The listing builds one solid part. Answer for the finished solid, in the listing's coordinates (mm). A direction names the side the tool comes from. Coordinates: 2 decimals unless noted, no trailing zeros. Order: outer loops, then holes, each group sorted by start corner. A loop starts at its lowest first (then second) coordinate and runs counter-clockwise, first axis right, second up. Notation, with made-up numbers: (54, 45) -> (59, 45) arc R35 ccw to (59, 79) -> close; hole circle Ø1 at (35, 3). An arc over 180 degrees is marked (long way). Answer in a Markdown table with one row per item.
```python
from build123d import *

# Parameters (mm, degrees)
EXTRUDE_2_DEPTH = 40


with BuildPart() as part:
    # 草图1 → 凸台-拉伸2 (new body)
    with BuildSketch(Plane(origin=(0, 0, 0), x_dir=(1, 0, 0), z_dir=(0, 1, 0))):
        with BuildLine():
            Line((1, 1), (1, 2.775338))
            ThreePointArc((1, 2.775338), (0, 2.95), (-1, 2.775338))
            Line((-1, 2.775338), (-1, 1))
            Line((-1, 1), (-2.775338, 1))
            ThreePointArc((-2.775338, 1), (-2.95, 0), (-2.775338, -1))
            Line((-2.775338, -1), (-1, -1))
            Line((-1, -1), (-1, -2.775338))
            ThreePointArc((-1, -2.775338), (0, -2.95), (1, -2.775338))
            Line((1, -2.775338), (1, -1))
            Line((1, -1), (2.775338, -1))
            ThreePointArc((2.775338, -1), (2.95, 0), (2.775338, 1))
            Line((2.775338, 1), (1, 1))
        make_face()
    extrude(amount=EXTRUDE_2_DEPTH)

    # 草图3 → 旋转3 (revolve)
    with BuildSketch(Plane(origin=(0, 0, 0), x_dir=(0, 0, -1), z_dir=(1, 0, 0))):
        with BuildLine():
            Line((0, 40), (0, 47))
            Line((0, 47), (2.95, 47))
            Line((2.95, 47), (2.95, 46))
            ThreePointArc((2.95, 46), (1.918246, 44.25), (2.95, 42.5))
            Line((2.95, 42.5), (2.95, 40))
            Line((2.95, 40), (0, 40))
        make_face()
        with BuildLine():
            Line((0, 0), (0, -7))
            Line((0, -7), (2.95, -7))
            Line((2.95, -7), (2.95, -6))
            ThreePointArc((2.95, -6), (1.918246, -4.25), (2.95, -2.5))
            Line((2.95, -2.5), (2.95, 0))
            Line((2.95, 0), (0, 0))
        make_face()
    revolve(axis=Axis((0, 0, 0), (0, -1, 0)))


solid = part.part
```
(1) A cutting plane is placed at A-A, the plane z = 0. Determine the outline of the cut face in (x, y), then the cut area to 3 significant figures.
Check values:
| item | result |
|---|---|
| outline | (-2.95, -7) -> (2.95, -7) -> (2.95, -6) arc R2 cw to (2.95, -2.5) -> (2.95, 42.5) arc R2 cw to (2.95, 46) -> (2.95, 47) -> (-2.95, 47) -> (-2.95, 46) arc R2 cw to (-2.95, 42.5) -> (-2.95, -2.5) arc R2 cw to (-2.95, -6) -> close |
| area | 308 mm² |
(2) Flat-ended cylindrical pins translate along their axes: pin 1 (0.9 mm diameter, centred on x = -1.5, y = 10, fed in from +Z); pin 2 (1 mm diameter, centred on y = -1.5, z = 1, fed in from -X); pin 3 (0.5 mm diameter, centred on y = 11.5, z = 2, fed in from -X). Find the tip coordinate at first contact, or state that the pin passes through.
Check values:
| item | result |
|---|---|
| pin 1 | z = 1 |
| pin 2 | x = -2.91 |
| pin 3 | x = -1 |
(3) For a pull along Y with two mould halves and no side action, classify faces 5 (the flat face through (0, 47, 0)), 6 (the flat face through (-1.7, 40, 1.7)), 7 (the flat face through (-1.7, 0, 1.7)), 8 (the cylindrical face through (0.13, -6.493, 2.947)) as released by +Y, released by -Y, zero draft, split by the parting line, or undercut.
Check values:
| item | result |
|---|---|
| face 5 | released by +Y |
| face 6 | undercut |
| face 7 | undercut |
| face 8 | zero draft |
(4) Find the intervals of material crossed by line 1 along Y through (x, z) = (1.7, -1.3); line 2 along Y through (x, z) = (-1.75, -1.75); line 3 along Z through (x, y) = (2.3, 14), in increasing order. Write a range as from..to.
Check values:
| item | result |
|---|---|
| line 1 | -7..-5.17, -3.33..0, 40..43.33, 45.17..47 |
| line 2 | -7..-5.63, -2.87..0, 40..42.87, 45.63..47 |
| line 3 | -1..1 |
(5) A cutting plane is placed at B-B, the plane x = 0. Determine the outline of the cut face in (y, z).
Check values:
| item | result |
|---|---|
| outline | (-7, -2.95) -> (-6, -2.95) arc R2 cw to (-2.5, -2.95) -> (42.5, -2.95) arc R2 cw to (46, -2.95) -> (47, -2.95) -> (47, 2.95) -> (46, 2.95) arc R2 cw to (42.5, 2.95) -> (-2.5, 2.95) arc R2 cw to (-6, 2.95) -> (-7, 2.95) -> close |
(6) A cutting plane is placed at C-C, the plane y = -2. Determine the outline of the cut face in (x, z), then the cut area to 3 significant figures.
Check values:
| item | result |
|---|---|
| outline | circle Ø5.9 at (0, 0) |
| area | 27.3 mm² |
(7) A cutting plane is placed at D-D, the plane z = 1.95. Count the separate pieces of the cut face and the enclosed holes in it, then the cut area to 3 significant figures.
Check values:
| item | result |
|---|---|
| separate pieces | 3 |
| enclosed holes | 0 |
| area | 123 mm² |
(8) Which of the six approach directions +Z, -Z, +X, -X, +Y, -Y give full straight-line access (tool end or side, diameter ignored) to faces 1 (the flat face through (1.7, 40, 1.7)), 2 (the flat face through (-1, 20, 2)), 3 (the flat face through (2, 20, -1)), 4 (the flat face through (-1.7, 40, -1.7))?
Check values:
| item | result |
|---|---|
| face 1 | +Z, +X |
| face 2 | +Z, -X |
| face 3 | -Z, +X |
| face 4 | -Z, -X |
